Read the model definition and answer for the solid it produces. Units are mm, in the model's axes. A direction names the side the tool comes from. Round coordinates to 2 decimals unless told otherwise and drop trailing zeros. Order: outer loops, then holes, each group sorted by start corner. A loop starts at its lowest first (then second) coordinate and runs counter-clockwise, first axis right, second up. Notation, with made-up numbers: (22.5, 63.25) -> (78.5, 63.25) arc R21 ccw to (78.5, 92.25) -> close; hole circle Ø4 at (28, -25). An arc over 180 degrees is marked (long way). Answer as a JSON object with one key per item and string values. Group by question number.
Item 1: The mould has two halves that part along Y. Classify faces 3 (the cylindrical face through (36.354, -13.955, 1.521)), 4 (the flat face through (-1, -25, 1)), 5 (the flat face through (-1, 25, 1)), 6 (the flat face through (0, 3.25, 2)): pulls with the +Y half, pulls with the -Y half, needs draft (parallel to the pull), parting line crosses it, or undercut.
Item 2: Section D-D, the plane z = 1.6 is taken. Count the separate pieces of the cut face and the enclosed holes in it, plus the area to 3 significant figures.
Item 3: Section A-A, the plane x = 0 is taken. Write down the section's boundary in (y, z).
Item 4: Consider probe 1 along Y at (x, z) = (1, 0.5); probe 2 along X at (y, z) = (-5.5, 2.75). Determine where each line is inside the solid, lowest interval first. Write a range as from..to.
Item 5: Section C-C, the plane x = 15 is taken. Write down the section's boundary in (y, z).
Item 6: For faces 1 (the cylindrical face through (-19.23, 4.255, 1.521)), 2 (the flat face through (-1, 0, 0)), determine the directions among +Z, -Z, +X, -X, +Y, -Y from which every point of the face is accessible in a straight line to the end or side of a thin tool.
Item 7: Given P1, Ø2.5, axis at x = 15, y = 0, coming from the -Z side; P2, Ø3.5, axis at x = -41, y = -18.5, coming from the -Z side, each flat-ended and moving along its own axis, determine where each tip first touches the part or whether it passes through.
Item 8: Section B-B, the plane y = -8.5 is taken. Write down the section's boundary in (x, z), plus the area to 3 significant figures.
from build123d import *

# Parameters (mm, degrees)
SKETCH1_W           = 95
SKETCH1_H           = 50
BOSS_EXTRUDE1_DEPTH = 3
SKETCH4_R           = 2
CUT_EXTRUDE3_DEPTH  = 4
SKETCH5_R           = 1.5
CUT_EXTRUDE4_DEPTH  = 4


with BuildPart() as part:
    # Sketch1 → Boss-Extrude1 (new body)
    with BuildSketch(Plane.XY):
        Rectangle(SKETCH1_W, SKETCH1_H)
    extrude(amount=BOSS_EXTRUDE1_DEPTH)

    # Sketch4 → Cut-Extrude3 (cut, through all)
    with BuildSketch(Plane.XY.offset(3)):
        with Locations((-15, 0)):
            Circle(SKETCH4_R)
        with Locations((15, 0)):
            Circle(SKETCH4_R)
        with Locations((-35, 0)):
            Circle(SKETCH4_R)
    extrude(amount=-CUT_EXTRUDE3_DEPTH, mode=Mode.SUBTRACT)

    # Sketch5 → Cut-Extrude4 (cut, through all)
    with BuildSketch(Plane.XY.offset(3)):
        with Locations((41, 18.5)):
            Circle(SKETCH5_R)
        with Locations((-41, 18.5)):
            Circle(SKETCH5_R)
        with BuildLine():
            Line((-34.5, 18.5), (-18.25, 18.5))
            Line((-18.25, 18.5), (-18.25, 5.04356025))
            ThreePointArc((-18.25, 5.04356025), (-19.242640687, 4.242640687), (-20.04356025, 3.25))
            Line((-20.04356025, 3.25), (-31.200328962, 3.25))
            ThreePointArc((-31.200328962, 3.25), (-35, 5), (-38.799671038, 3.25))
            Line((-38.799671038, 3.25), (-41, 3.25))
            Line((-41, 3.25), (-41, 12))
            ThreePointArc((-41, 12), (-36.403805922, 13.903805922), (-34.5, 18.5))
        make_face()
        with BuildLine():
            Line((-11.75, 5.04356025), (-11.75, 18.5))
            Line((-11.75, 18.5), (11.75, 18.5))
            Line((11.75, 18.5), (11.75, 5.04356025))
            ThreePointArc((11.75, 5.04356025), (10.757359313, 4.242640687), (9.95643975, 3.25))
            Line((9.95643975, 3.25), (-9.95643975, 3.25))
            ThreePointArc((-9.95643975, 3.25), (-10.757359313, 4.242640687), (-11.75, 5.04356025))
        make_face()
        with BuildLine():
            Line((18.25, 5.04356025), (18.25, 18.5))
            Line((18.25, 18.5), (34.5, 18.5))
            ThreePointArc((34.5, 18.5), (36.403805922, 13.903805922), (41, 12))
            Line((41, 12), (41, 3.25))
            Line((41, 3.25), (20.04356025, 3.25))
            ThreePointArc((20.04356025, 3.25), (19.242640687, 4.242640687), (18.25, 5.04356025))
        make_face()
    cut_extrude4 = extrude(amount=-CUT_EXTRUDE4_DEPTH, mode=Mode.SUBTRACT)

    # Mirror2: Cut-Extrude4 across plane
    add(cut_extrude4.mirror(Plane.ZX), mode=Mode.SUBTRACT)


solid = part.part
Values found:
{
 "1": {"face 3": "undercut", "face 4": "pulls with the -Y half", "face 5": "pulls with the +Y half", "face 6": "undercut"},
 "2": {"separate pieces": "1", "enclosed holes": "13", "area": "2,750 mm2"},
 "3": {"outline": "(-25, 0) -> (-18.5, 0) -> (-18.5, 3) -> (-25, 3) -> close; (-3.25, 0) -> (3.25, 0) -> (3.25, 3) -> (-3.25, 3) -> close; (18.5, 0) -> (25, 0) -> (25, 3) -> (18.5, 3) -> close"},
 "4": {"probe 1": "-25..-18.5, -3.25..3.25, 18.5..25", "probe 2": "-47.5..-41, -18.25..-11.75, 11.75..18.25, 41..47.5"},
 "5": {"outline": "(-25, 0) -> (-2, 0) -> (-2, 3) -> (-25, 3) -> close; (2, 0) -> (25, 0) -> (25, 3) -> (2, 3) -> close"},
 "6": {"face 1": "+Z, -Z", "face 2": "-Z, +X, -X, +Y, -Y"},
 "7": {"P1": "through", "P2": "z = 0"},
 "8": {"outline": "(-47.5, 0) -> (-41, 0) -> (-41, 3) -> (-47.5, 3) -> close; (-18.25, 0) -> (-11.75, 0) -> (-11.75, 3) -> (-18.25, 3) -> close; (11.75, 0) -> (18.25, 0) -> (18.25, 3) -> (11.75, 3) -> close; (41, 0) -> (47.5, 0) -> (47.5, 3) -> (41, 3) -> close", "area": "78.0 mm2"}
}
